from build123d import *

# Parameters (mm, degrees)
F0_W     = 22
F0_H     = 17
F0_W_2   = 20
F0_H_2   = 15
F1_DEPTH = 25
F2_R     = 2
F3_W     = 0.3
F3_H     = 1
F4_DEPTH = 3
F5_R     = 0.5


with BuildPart() as f1:
    # F0 (on Top) → F1 (new body)
    with BuildSketch(Plane.XY):
        with Locations((11, 8.5)):
            Rectangle(F0_W, F0_H)
        with Locations((11, 8.5)):
            Rectangle(F0_W_2, F0_H_2, mode=Mode.SUBTRACT)
    extrude(amount=F1_DEPTH)

    # F2
    f2_edges = [f1.edges().sort_by_distance(p)[0] for p in [
        (0, 17, 12.5),
        (0, 0, 12.5),
        (22, 0, 12.5),
        (22, 17, 12.5),
    ]]
    fillet(f2_edges, radius=F2_R)

    # F3 (on face) → F4 (cut)
    with BuildSketch(Plane(origin=(0, 0, 0), x_dir=(1, 0, 0), z_dir=(0, 0, -1))):
        with Locations((21.15, -8.5)):
            Rectangle(F3_W, F3_H)
    extrude(amount=-F4_DEPTH, mode=Mode.SUBTRACT)

    # F5
    f5_edges = [f1.edges().sort_by_distance(p)[0] for p in [
        (21, 1, 12.5),
        (1, 1, 12.5),
        (1, 16, 12.5),
        (21, 16, 12.5),
    ]]
    fillet(f5_edges, radius=F5_R)


solid = f1.part
Input: part model. Units: mm. Frame: model coordinates. A direction names the side the tool comes from. Coordinates: 2 decimals unless noted, no trailing zeros. Loops run counter-clockwise (first coordinate to the right, second up) from the corner with the lowest first, then second, coordinate; pieces in that order, holes last. Notation, with made-up numbers: (56.25, 58.5) -> (76.25, 58.5) arc R16 cw to (76.25, 88.5) -> close; hole circle Ø10 at (20.25, 55). An arc over 180 degrees is marked (long way). One line per item, written item: value.
(1) Cut plane C-C (x = 9.5). Output: boundary loops of the cut face in (y, z), then the cut area to 3 significant figures.
Answer below:
outline: (0, 0) -> (1, 0) -> (1, 25) -> (0, 25) -> close; (16, 0) -> (17, 0) -> (17, 25) -> (16, 25) -> close
area: 50.0 mm2
(2) Ray query, line 1 along X through (y, z) = (6.75, 14); line 2 along Y through (x, z) = (15, 2.5); line 3 along X through (y, z) = (1.5, 10.25). Return the intervals inside material, ascending.
Answer below:
line 1: x = 0 to 1, 21 to 22
line 2: y = 0 to 1, 16 to 17
line 3: x = 0.06 to 1, 21 to 21.94
(3) Cut plane A-A (y = 12). Output: boundary loops of the cut face in (x, z), then the cut area to 3 significant figures.
Answer below:
outline: (0, 0) -> (1, 0) -> (1, 25) -> (0, 25) -> close; (21, 0) -> (22, 0) -> (22, 25) -> (21, 25) -> close
area: 50.0 mm2
(4) Set-up query: faces 4 (the face through (21.4, 0.57, 12.68)), 5 (the face through (11, 16, 12)). Return all of +Z, -Z, +X, -X, +Y, -Y with unobstructed straight access to the full face (end or side cutting, diameter ignored); none if empty.
Answer below:
face 4: +Z, -Z, +X, -Y
face 5: +Z, -Z
(5) Cut plane B-B (z = 17.5). Output: boundary loops of the cut face in (x, y), then the cut area to 3 significant figures.
Answer below:
outline: (0, 2) arc R2 ccw to (2, 0) -> (20, 0) arc R2 ccw to (22, 2) -> (22, 15) arc R2 ccw to (20, 17) -> (2, 17) arc R2 ccw to (0, 15) -> close; hole (1, 1.5) arc R0.5 ccw to (1.5, 1) -> (20.5, 1) arc R0.5 ccw to (21, 1.5) -> (21, 15.5) arc R0.5 ccw to (20.5, 16) -> (1.5, 16) arc R0.5 ccw to (1, 15.5) -> close
area: 70.8 mm2
(6) Draft query along Y for faces 1 (the face through (21.3, 8.5, 1.5)), 2 (the face through (22, 8, 12)), 3 (the face through (11, 17, 12)). Return one class per face: pulls with the +Y half, pulls with the -Y half, needs draft (parallel to the pull), parting line crosses it, or undercut.
Answer below:
face 1: undercut
face 2: needs draft
face 3: pulls with the +Y half
